```python
from build123d import *

# Parameters (mm, degrees)
F2_W        = 3.175
F2_H        = 6.35
F3_DEPTH    = 9.525
F4_W        = 3.175
F4_H        = 0.9305988193
F5_DEPTH    = 25.4
F6_R        = 5.08
F7_T1_DEPTH = 27.9764149579
F7_T4_ANGLE = 90
F7_T6_ANGLE = 90
F9_R        = 6.35
F10_DEPTH   = 137.922
F11_R       = 7.62
F12_DEPTH   = 44.3738


# Not quite as in the source:
# - a fillet or chamfer that OpenCascade refuses, or shapes differently, is made with other operations: its cross-section is extruded or revolved along the edge and cut away or added
# - the program builds the solid bodies; features that only make, move or delete a surface that nothing else refers to are left out


with BuildPart() as f3:
    # F2 (on Top) → F3 (new body)
    with BuildSketch(Plane.XY):
        with Locations((0, 5.175651788)):
            Rectangle(F2_W, F2_H)
    extrude(amount=F3_DEPTH)

    # F4 (on face) → F5 (join)
    with BuildSketch(Plane(origin=(0, 8.350651788, 0), x_dir=(-1, 0, 0), z_dir=(0, 1, 0))):
        with Locations((0, 9.0597005904)):
            Rectangle(F4_W, F4_H)
    extrude(amount=F5_DEPTH)

    # F6
    f6_edges = [f3.edges().sort_by_distance(p)[0] for p in [
        (0, 8.350652, 8.594401),
        (0, 2.000652, 9.525),
    ]]
    fillet(f6_edges, radius=F6_R)

    # F7: chamfer of 0.508 on 2 edges, made by hand

    # F7_s2 → F7_t1 (cut)
    with BuildSketch(Plane.XZ.offset(-35.0570667459)):
        Polygon((1.5875, 9.017), (1.0795, 9.525), (1.5875, 9.525), align=None)
        Polygon((-1.5875, 9.017), (-1.0795, 9.525), (-1.5875, 9.525), align=None)
    extrude(amount=F7_T1_DEPTH, mode=Mode.SUBTRACT)

    # F7_s3 → F7_t4 (revolve, cut)
    with BuildSketch(Plane.XZ.offset(-7.080651788)):
        Polygon((-1.5875, 9.017), (-1.0795, 9.525), (-1.5875, 9.525), align=None)
    revolve(axis=Axis((-1.5875, 7.080651788, 4.445), (1, 0, 0)), revolution_arc=F7_T4_ANGLE, mode=Mode.SUBTRACT)

    # F7_s5 → F7_t6 (revolve, cut)
    with BuildSketch(Plane.XZ.offset(-7.080651788)):
        Polygon((1.5875, 9.017), (1.0795, 9.525), (1.5875, 9.525), align=None)
    revolve(axis=Axis((1.5875, 7.080651788, 4.445), (1, 0, 0)), revolution_arc=F7_T6_ANGLE, mode=Mode.SUBTRACT)

    # F9 (on Front) → F10 (join)
    with BuildSketch(Plane.XZ):
        Circle(F9_R)
    extrude(amount=-F10_DEPTH)

    # F11 (on face) → F12 (join)
    with BuildSketch(Plane.XZ.offset(-88.9)):
        Circle(F11_R)
    extrude(amount=-F12_DEPTH)


solid = f3.part
```
Check sheet for the modelled part. Datum: model origin and axes. Units: mm. A direction names the side the tool comes from. Round coordinates to 2 decimals unless told otherwise and drop trailing zeros. Order: outer loops, then holes, each group sorted by start corner. A loop starts at its lowest first (then second) coordinate and runs counter-clockwise, first axis right, second up.
1) Section check B-B (x = -4.25). Record the boundary of the cut face in (y, z), and give its area (3 significant figures).
2) Section check A-A (z = 0). Record the boundary of the cut face in (x, y), and give its area (3 significant figures).
3) Go/stop test with flat-tipped pins: pin 1 Ø6 at (x, y) = (-5.5, 92.5) entering from -Z; pin 2 Ø0.9 at (y, z) = (25, 8) entering from -X; pin 3 Ø1 at (x, y) = (-1.5, 52) entering from +Z; pin 4 Ø1 at (x, y) = (0.5, 26) entering from -Z. Record where each tip stops, or that it passes through.
4) Section check C-C (y = 49.5). Record the boundary of the cut face in (x, z).
5) Tool access check on faces 1 (the flat face through (1.588, 12.5, 8.85)), 2 (the flat face through (0, 0, 0)), 3 (the flat face through (-3, 133.274, 6)), 4 (the flat face through (-1.588, 12.5, 8.85)), 5 (the flat face through (0, 23, 8.594)). Record the directions out of +Z, -Z, +X, -X, +Y, -Y that give a thin tool (end or side, any length) a straight path to the whole face; none if there is none.
6) Scan lines: line 1 (Y direction, x = -6, z = 4); line 2 (Z direction, x = 1.5, y = 22.5); line 3 (X direction, y = 39, z = 4.5). Record each from-to range of solid material in increasing order.
Result:
1. outline: (0, -4.72) - (88.9, -4.72) - (88.9, -6.32) - (133.27, -6.32) - (133.27, -4.72) - (137.92, -4.72) - (137.92, 4.72) - (133.27, 4.72) - (133.27, 6.32) - (88.9, 6.32) - (88.9, 4.72) - (0, 4.72) - close
1. area: 1,440 mm2
2. outline: (-7.62, 88.9) - (-6.35, 88.9) - (-6.35, 0) - (6.35, 0) - (6.35, 88.9) - (7.62, 88.9) - (7.62, 133.27) - (6.35, 133.27) - (6.35, 137.92) - (-6.35, 137.92) - (-6.35, 133.27) - (-7.62, 133.27) - close
2. area: 1,860 mm2
3. pin 1: stops at z = -7.2
3. pin 2: passes through
3. pin 3: stops at z = 6.27
3. pin 4: stops at z = -6.35
4. outline: circle Ø12.7 at (0, 0)
5. face 1: +Z, +X, -Y
5. face 2: +Z, -Z, +X, -X, -Y
5. face 3: +Y
5. face 4: +Z, -X, -Y
5. face 5: +X, -X, +Y
6. line 1: y = 88.9 to 133.27
6. line 2: z = -6.17 to 6.17, 8.59 to 9.1
6. line 3: x = -4.48 to 4.48
